For this review, take the finished solid that the model builds, in its own axes (mm). A direction names the side the tool comes from. Round coordinates to 2 decimals unless told otherwise and drop trailing zeros. Loops run counter-clockwise (first coordinate to the right, second up) from the corner with the lowest first, then second, coordinate; pieces in that order, holes last.
1) Take a section at D-D (x = -40.5). State the section outline as (y, z) points, then the cut area to 3 significant figures.
2) Take a section at B-B (x = 0). State the section outline as (y, z) points, then the cut area to 3 significant figures.
3) Insertion check: pin 1 (6 mm diameter, centred on x = -39.5, z = 0.5, fed in from +Y); pin 2 (1.6 mm diameter, centred on x = -1, z = -41, fed in from +Y). Each pin has a flat end and moves straight along its axis. Give the tip position at first contact, or say it passes through.
4) Tool access review of faces 1 (the cylindrical face through (-0.34, 2.1, -43.13)), 2 (the flat face through (-1, 0, -1)): name each direction out of +Z, -Z, +X, -X, +Y, -Y from which nothing blocks a thin tool from reaching the whole face with its end or side.
5) Take a section at C-C (z = 40.5). State the section outline as (x, y) points, then the cut area to 3 significant figures.
6) Wall thickness on L1, parallel to Z at x = 0, y = 5.15; L2, parallel to X at y = 2.9, z = -40.5: over which ranges is each line inside the solid? List them lowest first.
7) Mouldability with a two-part tool opening along Z and no side actions: class faces 3 (the cylindrical face through (-10.12, 5.27, 45.59)), 4 (the flat face through (-77, 3, 1)), 5 (the flat face through (-1, 3, -77)) as pulls with the +Z half, pulls with the -Z half, needs draft (parallel to the pull), parting line crosses it, or undercut.
8) Take a section at A-A (z = 0). State the section outline as (x, y) points, then the cut area to 3 significant figures.
```python
from build123d import *

# Parameters (mm, degrees)
SKETCH1_W           = 154
SKETCH1_H           = 154
BOSS_EXTRUDE1_DEPTH = 6.5
SKETCH2_R           = 46.7
CUT_EXTRUDE1_DEPTH  = 2.5
SKETCH3_R           = 2.65
CUT_EXTRUDE2_DEPTH  = 3.5
CHAMFER1_SIZE       = 0.2
CHAMFER1_SIZE2      = 0.346410162


with BuildPart() as part:
    # Sketch1 → Boss-Extrude1 (new body)
    with BuildSketch(Plane(origin=(0, 0, 0), x_dir=(1, 0, 0), z_dir=(0, 1, 0))):
        Rectangle(SKETCH1_W, SKETCH1_H)
    extrude(amount=BOSS_EXTRUDE1_DEPTH)

    # Sketch2 → Cut-Extrude1 (cut)
    with BuildSketch(Plane(origin=(0, 6.5, 0), x_dir=(1, 0, 0), z_dir=(0, 1, 0))):
        Circle(SKETCH2_R)
    extrude(amount=-CUT_EXTRUDE1_DEPTH, mode=Mode.SUBTRACT)

    # Sketch3 → Cut-Extrude2 (cut)
    with BuildSketch(Plane(origin=(0, 4, 0), x_dir=(1, 0, 0), z_dir=(0, 1, 0))):
        with Locations((0, 40.5)):
            Circle(SKETCH3_R)
        with Locations((-40.5, 0)):
            Circle(SKETCH3_R)
        with Locations((0, -40.5)):
            Circle(SKETCH3_R)
        with Locations((40.5, 0)):
            Circle(SKETCH3_R)
    extrude(amount=-CUT_EXTRUDE2_DEPTH, mode=Mode.SUBTRACT)

    # Chamfer1
    chamfer1_edges = [part.edges().sort_by_distance(p)[0] for p in [
        (-2.65, 4, -40.5),
        (-43.15, 4, 0),
        (-2.65, 4, 40.5),
        (37.85, 4, 0),
    ]]
    chamfer1_side = [part.faces().sort_by_distance(p)[0] for p in [
        (0, 4, 0),
    ]]
    chamfer(chamfer1_edges, length=CHAMFER1_SIZE, length2=CHAMFER1_SIZE2, reference=chamfer1_side[0])


solid = part.part
```
Response:
1. outline: (0, -77) - (6.5, -77) - (6.5, -23.25) - (4, -23.25) - (4, -2.85) - (3.65, -2.65) - (0.5, -2.65) - (0.5, 2.65) - (3.65, 2.65) - (4, 2.85) - (4, 23.25) - (6.5, 23.25) - (6.5, 77) - (0, 77) - close
1. area: 866 mm2
2. outline: (0, -77) - (6.5, -77) - (6.5, -46.7) - (4, -46.7) - (4, -43.35) - (3.65, -43.15) - (0.5, -43.15) - (0.5, -37.85) - (3.65, -37.85) - (4, -37.65) - (4, 37.65) - (3.65, 37.85) - (0.5, 37.85) - (0.5, 43.15) - (3.65, 43.15) - (4, 43.35) - (4, 46.7) - (6.5, 46.7) - (6.5, 77) - (0, 77) - close
2. area: 730 mm2
3. pin 1: stops at y = 4
3. pin 2: stops at y = 0.5
4. face 1: +Y
4. face 2: +Z, -Z, +X, -X, -Y
5. outline: (-77, 0) - (77, 0) - (77, 6.5) - (23.25, 6.5) - (23.25, 4) - (2.85, 4) - (2.65, 3.65) - (2.65, 0.5) - (-2.65, 0.5) - (-2.65, 3.65) - (-2.85, 4) - (-23.25, 4) - (-23.25, 6.5) - (-77, 6.5) - close
5. area: 866 mm2
6. L1: z = -77 to -46.7, 46.7 to 77
6. L2: x = -77 to -2.65, 2.65 to 77
7. face 3: undercut
7. face 4: needs draft
7. face 5: pulls with the -Z half
8. outline: (-77, 0) - (77, 0) - (77, 6.5) - (46.7, 6.5) - (46.7, 4) - (43.35, 4) - (43.15, 3.65) - (43.15, 0.5) - (37.85, 0.5) - (37.85, 3.65) - (37.65, 4) - (-37.65, 4) - (-37.85, 3.65) - (-37.85, 0.5) - (-43.15, 0.5) - (-43.15, 3.65) - (-43.35, 4) - (-46.7, 4) - (-46.7, 6.5) - (-77, 6.5) - close
8. area: 730 mm2
